For this review, use the dimensioned drawing (mm, ordinates from the lowest corner) and the shaded views. Round coordinates to 2 decimals unless told otherwise and drop trailing zeros. Write each loop counter-clockwise with the first axis right and the second up, starting at its lowest first coordinate (ties: lowest second). Pieces come first, ordered by that corner, then holes. Notation, with made-up numbers: M -16,4 L -12,4 A14 ccw -12,28 Z; hole C 85.5,86 d5. An arc over 180 degrees is marked long. Use CSV: the item, a comma, the result in double quotes.
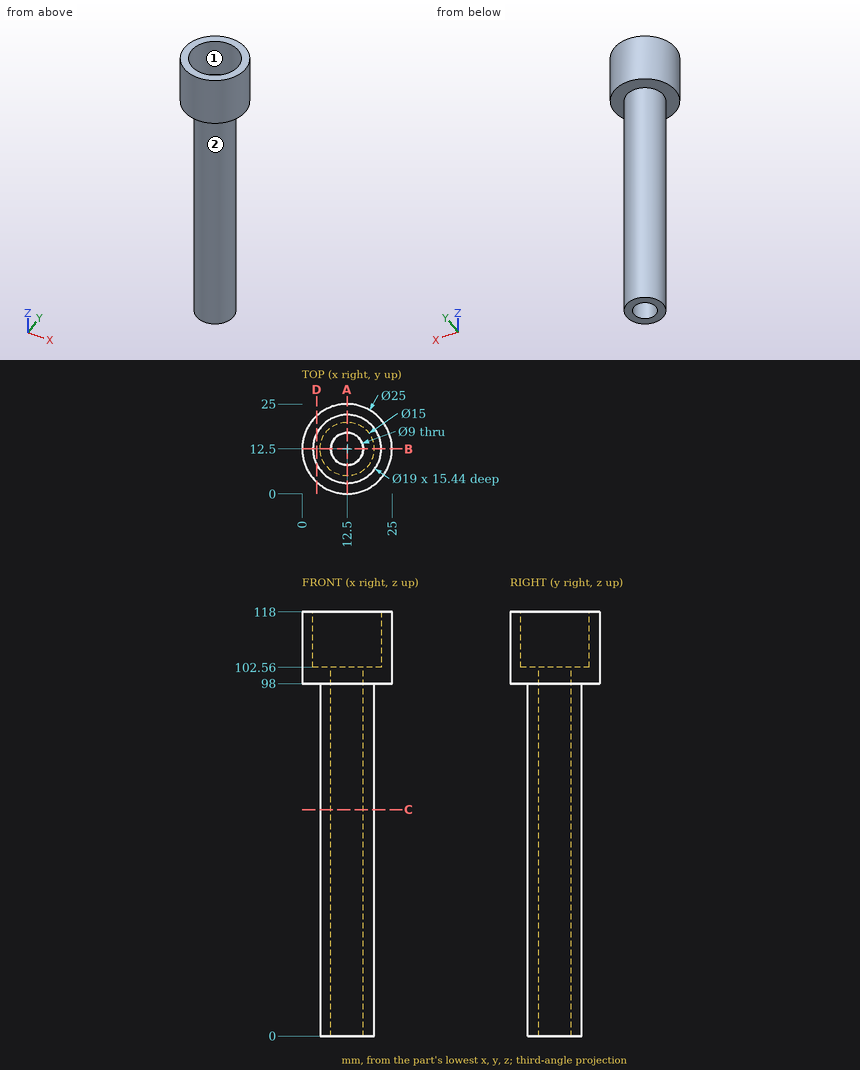
1) Add section C-C on z = 63. Write out the cut boundary in (x, y).
Answers:
outline,"C 12.5,12.5 d15; hole C 12.5,12.5 d9"
2) Add section D-D on x = 4. Write out the cut boundary in (y, z), then the cut area to 3 significant figures.
Answers:
outline,"M 3.33,98 L 21.67,98 L 21.67,118 L 16.74,118 L 16.74,102.56 L 8.26,102.56 L 8.26,118 L 3.33,118 Z"
area,"236 mm²"
3) Wall thickness on line 1 along Y through (x, z) = (12.5, 110.75); line 2 along Y through (x, z) = (12.5, 42); line 3 along Z through (x, y) = (11.75, 3.75): over which ranges is each line inside the solid? List them lowest first. Write a range as [from, to].
Answers:
line 1,"[0, 3], [22, 25]"
line 2,"[5, 8], [17, 20]"
line 3,"[98, 102.56]"
4) For pin 1 Ø3 at (x, z) = (10.5, 95.5) entering from -Y; pin 2 Ø1 at (x, y) = (20.5, 4) entering from -Z; pin 3 Ø5 at (y, z) = (14.5, 74) entering from +X; pin 4 Ø3 at (x, z) = (22.5, 47.5) entering from -Y, all flat-tipped, find the tip position at first contact; note any pin that passes through.
Answers:
pin 1,"y = 5.02"
pin 2,"z = 98"
pin 3,"x = 20"
pin 4,"through"
5) Add section A-A on x = 12.5. Write out the cut boundary in (y, z).
Answers:
outline,"M 0,98 L 5,98 L 5,0 L 8,0 L 8,102.56 L 3,102.56 L 3,118 L 0,118 Z; M 17,0 L 20,0 L 20,98 L 25,98 L 25,118 L 22,118 L 22,102.56 L 17,102.56 Z"
6) The part is to be moulded in two halves that separate along X. For the marked faces 1 and 2, say which applies: released by +X, released by -X, zero draft, split by the parting line, or undercut.
Answers:
face 1,"undercut"
face 2,"split by the parting line"
